from build123d import *

# Parameters (mm, degrees)
F1_DEPTH = 25.4
F3_D     = 5.1054
F4_R     = 5.08
F5_R     = 5.08


with BuildPart() as f1:
    # F0 (on Front) → F1 (new body)
    with BuildSketch(Plane.XZ):
        with BuildLine():
            Line((19.05, 0), (19.05, 52.9124252498))
            ThreePointArc((19.05, 52.9124252498), (0, 71.9624252498), (-19.05, 52.9124252498))
            Line((-19.05, 52.9124252498), (-19.05, 0))
            Line((-19.05, 0), (19.05, 0))
        make_face()
    extrude(amount=F1_DEPTH)

    # F3 (through all)
    with Locations(Plane.XZ.offset(25.4)):
        with Locations((-11.1125, 44.45), (11.1125, 44.45), (11.1125, 19.05), (-11.1125, 19.05)):
            Hole(F3_D / 2)

    # F4
    f4_edges = [f1.edges().sort_by_distance(p)[0] for p in [
        (-19.05, -12.7, 0),
        (19.05, -12.7, 0),
    ]]
    fillet(f4_edges, radius=F4_R)

    # F5
    f5_edges = [f1.edges().sort_by_distance(p)[0] for p in [
        (-19.05, -25.4, 28.996213),
        (0, -25.4, 0),
        (0, 0, 0),
        (19.05, 0, 28.996213),
    ]]
    fillet(f5_edges, radius=F5_R)


solid = f1.part
Input: part model. Units: mm. Frame: model coordinates. Give positions to 0.01 mm unless a question says otherwise; leave off trailing zeros. Order: outer loops, then holes, each group sorted by start corner. A loop starts at its lowest first (then second) coordinate and runs counter-clockwise, first axis right, second up. Notation, with made-up numbers: (-17.75, 73) -> (32.25, 73) arc R8 cw to (32.25, 81) -> close; hole circle Ø6 at (-10.75, -26). An arc over 180 degrees is marked (long way). Use one line per item in the form item = value.
1) Mould query, pull axis X, two halves, no side actions, for faces 1 (the cylindrical face through (-17.522, -1.449, 28.661)), 2 (the cylindrical face through (-12.29, -12.522, 16.785)), 3 (the cylindrical face through (0.196, -23.951, 1.528)). Classes: pulls with the +X half, pulls with the -X half, needs draft (parallel to the pull), parting line crosses it, or undercut.
Response values:
face_1 = pulls with the -X half
face_2 = undercut
face_3 = needs draft
2) Section B-B, the plane z = 19.05. Return loops of the section in (x, y).
Response values:
outline = (-19.05, -20.32) arc R5.08 ccw to (-13.97, -25.4) -> (-13.67, -25.4) -> (-13.67, 0) -> (-13.97, 0) arc R5.08 ccw to (-19.05, -5.08) -> close; (-8.56, -25.4) -> (8.56, -25.4) -> (8.56, 0) -> (-8.56, 0) -> close; (13.67, -25.4) -> (13.97, -25.4) arc R5.08 ccw to (19.05, -20.32) -> (19.05, -5.08) arc R5.08 ccw to (13.97, 0) -> (13.67, 0) -> close
3) Line query: probe 1 along Z at (x, y) = (-10, -15.75); probe 2 along Z at (x, y) = (9, -14); probe 3 along Z at (x, y) = (-17, -7.75). Output: solid intervals per line, ascending.
Response values:
probe_1 = 0 to 16.75, 21.35 to 42.15, 46.75 to 69.13
probe_2 = 0 to 17.62, 20.48 to 43.02, 45.88 to 69.7
probe_3 = 1 to 61.51
4) Section D-D, the plane z = 43.5. Return loops of the section in (x, y), and give its area (3 significant figures).
Response values:
outline = (-19.05, -20.32) arc R5.08 ccw to (-13.97, -25.4) -> (-13.48, -25.4) -> (-13.48, 0) -> (-13.97, 0) arc R5.08 ccw to (-19.05, -5.08) -> close; (-8.74, -25.4) -> (8.74, -25.4) -> (8.74, 0) -> (-8.74, 0) -> close; (13.48, -25.4) -> (13.97, -25.4) arc R5.08 ccw to (19.05, -20.32) -> (19.05, -5.08) arc R5.08 ccw to (13.97, 0) -> (13.48, 0) -> close
area = 705 mm^2
5) First-contact query: pin 1 Ø8 at (y, z) = (-4.5, 8.5) entering from +X; pin 2 Ø4 at (x, y) = (-8, -8.5) entering from +Z. Flat tips, straight axial feed; report the tip coordinate or a pass-through.
Response values:
pin_1 = 19.05
pin_2 = 70.99
6) Section C-C, the plane y = -23.75. Return loops of the section in (x, z).
Response values:
outline = (-17.72, 5.08) arc R3.75 ccw to (-13.97, 1.33) -> (13.97, 1.33) arc R3.75 ccw to (17.72, 5.08) -> (17.72, 52.91) arc R17.72 ccw to (-17.72, 52.91) -> close; hole circle Ø5.11 at (-11.11, 19.05); hole circle Ø5.11 at (-11.11, 44.45); hole circle Ø5.11 at (11.11, 19.05); hole circle Ø5.11 at (11.11, 44.45)
7) Section A-A, the plane y = -7. Return loops of the section in (x, z).
Response values:
outline = (-19.05, 5.08) arc R5.08 ccw to (-13.97, 0) -> (13.97, 0) arc R5.08 ccw to (19.05, 5.08) -> (19.05, 52.91) arc R19.05 ccw to (-19.05, 52.91) -> close; hole circle Ø5.11 at (-11.11, 19.05); hole circle Ø5.11 at (-11.11, 44.45); hole circle Ø5.11 at (11.11, 19.05); hole circle Ø5.11 at (11.11, 44.45)
